```python
from build123d import *

# Parameters (mm, degrees)
SKETCH1_R           = 13
SKETCH1_R_2         = 1.1
BOSS_EXTRUDE1_DEPTH = 10
BOSS_EXTRUDE2_START = -3
SKETCH1_4_R         = 13
BOSS_EXTRUDE2_DEPTH = 3
FILLET1_R           = 3
SKETCH4_W           = 5.7
SKETCH4_H           = 5.7
CUT_EXTRUDE1_DEPTH  = 9
CIRPATTERN1_COUNT   = 5


with BuildPart() as part:
    # Sketch1 → Boss-Extrude1 (new body)
    with BuildSketch(Plane.XY):
        Circle(SKETCH1_R)
        Circle(SKETCH1_R_2, mode=Mode.SUBTRACT)
    extrude(amount=BOSS_EXTRUDE1_DEPTH)

    # Sketch1_4 → Boss-Extrude2 (add)
    with BuildSketch(Plane.XY.offset(BOSS_EXTRUDE2_START)):
        Circle(SKETCH1_4_R)
    extrude(amount=BOSS_EXTRUDE2_DEPTH)

    # Fillet1
    fillet1_edges = [part.edges().sort_by_distance(p)[0] for p in [
        (-13, 0, -3),
    ]]
    fillet(fillet1_edges, radius=FILLET1_R)

    # Sketch4 → Cut-Extrude1 (cut)
    with BuildSketch(Plane(origin=(-11.286443879, -6.451305765, 0), x_dir=(0.499999999999998, -0.8660254037844398, 0), z_dir=(0.8660254037844398, 0.499999999999998, 0))):
        with Locations((0.056227259, -3.15)):
            Rectangle(SKETCH4_W, SKETCH4_H)
    cut_extrude1 = extrude(amount=CUT_EXTRUDE1_DEPTH, mode=Mode.SUBTRACT)

    # CirPattern1: Cut-Extrude1 ×5 about axis
    cirpattern1_axis = Axis((0, 0, 0), (0, 0, 1))
    for i in range(1, CIRPATTERN1_COUNT):
        add(cut_extrude1.rotate(cirpattern1_axis, i * 360 / CIRPATTERN1_COUNT), mode=Mode.SUBTRACT)


solid = part.part
```
Here's how the part is built. I have some questions about the finished solid (model axes, mm). A direction names the side the tool comes from. Round coordinates to 2 decimals unless told otherwise and drop trailing zeros. Loops run counter-clockwise (first coordinate to the right, second up) from the corner with the lowest first, then second, coordinate; pieces in that order, holes last.
1. Thinking about a two-plate mould opening in Y: for faces 1 (the face through (3, 0, 10)), 2 (the face through (6.021, 6.517, 3.19)), 3 (the face through (5.999, -11.533, 4.93)), 4 (the face through (1.05, 0.33, 4.93)), which applies, released by +Y, released by -Y, zero draft, split by the parting line, or undercut?
Answers:
face 1: zero draft
face 2: released by +Y
face 3: split by the parting line
face 4: undercut
2. If I drill on probe 1 along Z at (x, y) = (4.5, 1.75); probe 2 along Y at (x, z) = (0, 3.25); probe 3 along Y at (x, z) = (0, 7.75), over which ranges is the centre line in solid material (lowest first)?
Answers:
probe 1: z = -3 to 0.3, 6 to 10
probe 2: y = -4.09 to -1.1, 1.1 to 4.38, 7.01 to 13
probe 3: y = -13 to -1.1, 1.1 to 13
3. Suppose I cut it at C-C, the plane z = -1.5. Please give me the cut outline in (x, y).
Answers:
outline: circle Ø25.2 at (0, 0)
4. Suppose I cut it at D-D, the plane z = 8. Please give me the cut outline in (x, y).
Answers:
outline: circle Ø26 at (0, 0); hole circle Ø2.2 at (0, 0)
5. Suppose I cut it at B-B, the plane y = 0. Please give me the cut outline in (x, z), and give its area (3 significant figures).
Answers:
outline: (-13, 0) arc R3 ccw to (-10, -3) - (10, -3) arc R3 ccw to (13, 0) - (13, 0.3) - (4.02, 0.3) - (4.02, 6) - (13, 6) - (13, 10) - (1.1, 10) - (1.1, 0) - (-1.1, 0) - (-1.1, 10) - (-13, 10) - close; hole (-5.7, 0.3) - (-4.62, 0.3) - (-4.62, 6) - (-5.7, 6) - close
area: 255 mm2
6. Will these pins go through, and if not, where does the flat tip stop? pin 1 (3 mm diameter, centred on y = -3.5, z = 5, fed in from -X); pin 2 (4 mm diameter, centred on x = 6.5, z = 5, fed in from +Y); pin 3 (0.7 mm diameter, centred on x = 0.5, y = -0.5, fed in from +Z).
Answers:
pin 1: stops at x = -12.85
pin 2: stops at y = 12.09
pin 3: stops at z = 0
7. Suppose I cut it at A-A, the plane z = 5. Please give me the cut outline in (x, y), and give its area (3 significant figures).
Answers:
outline: (-12.41, -3.87) - (-4.89, 0.47) - (-2.04, -4.47) - (-9.56, -8.81) arc R13 ccw to (-0.15, -13) - (-1.96, -4.51) - (3.62, -3.32) - (5.42, -11.81) arc R13 ccw to (12.32, -4.16) - (3.68, -3.25) - (4.28, 2.42) - (12.91, 1.51) arc R13 ccw to (7.76, 10.43) - (4.23, 2.49) - (-0.98, 4.81) - (2.56, 12.75) arc R13 ccw to (-7.52, 10.61) - (-1.07, 4.79) - (-4.88, 0.56) - (-11.33, 6.37) arc R13 ccw to start; hole circle Ø2.2 at (0, 0)
area: 274 mm2
8. For faces 5 (the face through (8.059, -3.713, 3.19)), 6 (the face through (0.79, -3.92, 3.11)), 7 (the face through (0, 0, -3)), which set-ups out of +Z, -Z, +X, -X, +Y, -Y let a thin tool reach every point of the face, with its end or its side?
Answers:
face 5: +X
face 6: none
face 7: -Z, +X, -X, +Y, -Y
